Autodesk Inventor part; units mm, degrees
ref_plane "YZ Plane" through (0, 0, 0) normal (1, 0, 0) x (0, 1, 0)
ref_plane "XZ Plane" through (0, 0, 0) normal (0, 1, 0) x (-1, 0, 0)
ref_plane "XY Plane" through (0, 0, 0) normal (0, 0, 1) x (1, 0, 0)
sketch "Sketch1" plane through (0, 0, 0) normal (0, 0, 1) x (1, 0, 0)
  line L0 (-160, -190) -> (160, -190)
  line L1 (160, -190) -> (160, 190)
  line L2 (160, 190) -> (-160, 190)
  line L3 (-160, 190) -> (-160, -190)
  line L4 (-160, -190) -> (160, 190) construction
  line L5 (160, -190) -> (-160, 190) construction
  point P0 (0, 0)
  dimension "d0" = 320
  dimension "d1" = 380
extrude "Extrusion1" add sketch "Sketch1" along normal blind 25
sketch "Sketch2" plane through (0, 0, 25) normal (0, 0, 1) x (1, 0, 0)
  line L0 (-37.5, -150) -> (37.5, -150) construction
  line L1 (37.5, -150) -> (37.5, 150) construction
  line L2 (37.5, 150) -> (-37.5, 150) construction
  line L3 (-37.5, 150) -> (-37.5, -150) construction
  line L4 (-37.5, -150) -> (37.5, 150) construction
  line L5 (37.5, -150) -> (-37.5, 150) construction
  point P0 (0, 0)
  point P1 (-37.5, 50)
  point P2 (37.5, 50)
  point P3 (-37.5, -50)
  point P4 (37.5, -50)
  dimension "d4" = 75
  dimension "d5" = 300
  dimension "d6" = 100
  dimension "d7" = 100
  dimension "d8" = 100
hole "Hole1" at (-37.5, 150, 25) at (37.5, 150, 25) at (-37.5, 50, 25) at (37.5, 50, 25) at (-37.5, -50, 25) at (37.5, -50, 25) at (-37.5, -150, 25) at (37.5, -150, 25) direction (0, 0, -1) diameter 5.134 end through all
chamfer "Chamfer1" distance 0.5 angle 45 8 edges at (-37.5, -147.433, 25) (-37.5, -47.433, 25) (37.5, -147.433, 25) (37.5, -47.433, 25) (-37.5, 52.567, 25) (-37.5, 152.567, 25) (37.5, 52.567, 25) (37.5, 152.567, 25)
sketch "Sketch5" plane through (0, 0, 25) normal (0, 0, 1) x (1, 0, 0)
  circle A0 centre (37.5, -150) radius 3.067 construction
  circle A1 centre (-37.5, -50) radius 3.067 construction
  circle A2 centre (-37.5, 50) radius 3.067 construction
  circle A3 centre (-37.5, 150) radius 3.067 construction
  line L0 (160, -190) -> (160, 190) construction
  line L1 (160, 190) -> (-160, 190) construction
  line L2 (-160, 190) -> (-160, -190) construction
  line L3 (-160, -190) -> (160, -190) construction
  circle A4 centre (37.5, 150) radius 3.067 construction
  circle A5 centre (37.5, 50) radius 3.067 construction
  circle A6 centre (37.5, -50) radius 3.067 construction
  circle A7 centre (-37.5, -150) radius 3.067 construction
  line L4 (146, 190) -> (146, -190) construction
  line L5 (160, -190) -> (160, 190)
  line L6 (160, 190) -> (-160, 190)
  line L7 (-160, -190) -> (160, -190)
  line L8 (0, 190) -> (0, -190) construction
  point P0 (0, 0)
  point P1 (146, 160)
  point P2 (146, 80)
  point P3 (146, 0)
  point P4 (146, -80)
  point P5 (146, -160)
  point P6 (-146, 160)
  point P7 (-146, 80)
  point P8 (-146, 0)
  point P9 (-146, -80)
  point P10 (-146, -160)
  dimension "d49" = 14
  dimension "d50" = 80
  dimension "d51" = 80
  dimension "d52" = 80
  dimension "d53" = 30
  dimension "d54" = 80
  dimension "d55" = 30
hole "Hole4" at (146, 160, 25) at (146, 80, 25) at (146, 0, 25) at (146, -80, 25) at (146, -160, 25) at (-146, 160, 25) at (-146, 80, 25) at (-146, 0, 25) at (-146, -80, 25) at (-146, -160, 25) direction (0, 0, -1) diameter 10.5 end through all counterbore diameter 18 counterbore depth 11
sketch "Sketch3" plane through (160, -190, 0) normal (1, 0, 0) x (0, 0, -1)
  line L0 (0, 380) -> (-25, 380) construction
  line L1 (-12.5, 380) -> (-12.5, 0) construction
  line L2 (0, 0) -> (-25, 0) construction
  point P0 (0, 190)
  point P1 (-12.5, 315)
  point P2 (-12.5, 250)
  point P3 (-12.5, 185)
  point P4 (-12.5, 120)
  point P5 (-12.5, 55)
  dimension "d19" = 65
  dimension "d20" = 65
  dimension "d21" = 65
  dimension "d22" = 65
  dimension "d25" = 65
  dimension "d26" = 55
sketch "Sketch4" plane through (-160, -190, 0) normal (-1, 0, 0) x (0, 0, 1)
  line L0 (0, 380) -> (25, 380) construction
  line L1 (12.5, 380) -> (12.5, 0) construction
  line L2 (0, 0) -> (25, 0) construction
  line L3 (0, 380) -> (25, 380)
  point P0 (0, 190)
  point P1 (12.5, 55)
  point P2 (12.5, 315)
  point P3 (12.5, 250)
  point P4 (12.5, 185)
  point P5 (12.5, 120)
  dimension "d37" = 65
  dimension "d38" = 65
  dimension "d39" = 65
  dimension "d40" = 65
  dimension "d41" = 65
properties part number "KN-00-01-03" material "X5CrNi18-10"
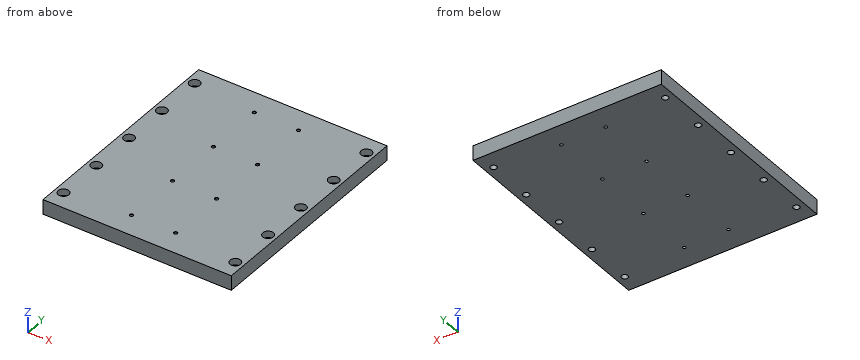
Build history of the part. All positions in model axes, mm. Coordinates: 2 decimals unless noted, no trailing zeros. Write each loop counter-clockwise with the first axis right and the second up, starting at its lowest first coordinate (ties: lowest second). Pieces come first, ordered by that corner, then holes.
(1) Cut at B-B on z = 19. State how many separate pieces and enclosed holes the cut face has, and give its area (3 significant figures).
(2) Cut at A-A on y = -80. List the corners of the cut face in (x, z), and give its area (3 significant figures).
(3) Drill centre lines: line 1 (Y direction, x = -146, z = 8.5); line 2 (Y direction, x = -37.5, z = 6.25); line 3 (Y direction, x = 146, z = 17.5). Where is each one in solid material? Low to high.
(4) Pin check, flat tips, straight feed: pin 1 Ø6 at (x, y) = (37.5, -50) entering from +Z; pin 2 Ø6.5 at (x, y) = (-146, 160) entering from -Z; pin 3 Ø14.5 at (x, y) = (146, -80) entering from -Z; pin 4 Ø5.5 at (x, y) = (147.5, 84) entering from +Z. Stop position of each tip, or through.
Working result:
1. separate pieces: 1
1. enclosed holes: 18
1. area: 119,000 mm2
2. outline: (-160, 0) - (-151.25, 0) - (-151.25, 14) - (-155, 14) - (-155, 25) - (-160, 25) - close; (-140.75, 0) - (140.75, 0) - (140.75, 14) - (137, 14) - (137, 25) - (-137, 25) - (-137, 14) - (-140.75, 14) - close; (151.25, 0) - (160, 0) - (160, 25) - (155, 25) - (155, 14) - (151.25, 14) - close
2. area: 7,310 mm2
3. line 1: y = -190 to -165.25, -154.75 to -85.25, -74.75 to -5.25, 5.25 to 74.75, 85.25 to 154.75, 165.25 to 190
3. line 2: y = -190 to -152.57, -147.43 to -52.57, -47.43 to 47.43, 52.57 to 147.43, 152.57 to 190
3. line 3: y = -190 to -169, -151 to -89, -71 to -9, 9 to 71, 89 to 151, 169 to 190
4. pin 1: stops at z = 24.93
4. pin 2: passes through
4. pin 3: stops at z = 0
4. pin 4: stops at z = 14
